Verification items for the finished model (mm, model axes). A direction names the side the tool comes from. Coordinates: 2 decimals unless noted, no trailing zeros. Write each loop counter-clockwise with the first axis right and the second up, starting at its lowest first coordinate (ties: lowest second). Pieces come first, ordered by that corner, then holes.
```python
from build123d import *

# Parameters (mm, degrees)
BOSS_EXTRUDE1_DEPTH = 1.7
BOSS_EXTRUDE4_DEPTH = 0.3
SKETCH6_R           = 1.45
CUT_EXTRUDE1_DEPTH  = 2
SKETCH7_R           = 1.45
CUT_EXTRUDE2_DEPTH  = 2
SKETCH8_R           = 0.25
CUT_EXTRUDE3_DEPTH  = 2
SKETCH9_R           = 0.25
CUT_EXTRUDE4_DEPTH  = 2


with BuildPart() as part:
    # Sketch1 → Boss-Extrude1 (new body)
    with BuildSketch(Plane.XY):
        Polygon((-93.349083219, 17.192602894), (-83.349083219, 17.192602894), (-83.349083219, 20.192602894), (-78.349083219, 20.192602894), (-78.349083219, 6.092602894), (-83.349083219, 6.092602894), (-83.349083219, 9.092602894), (-93.349083219, 9.092602894), (-93.349083219, 6.092602894), (-98.349083219, 6.092602894), (-98.349083219, 20.192602894), (-93.349083219, 20.192602894), align=None)
    extrude(amount=BOSS_EXTRUDE1_DEPTH)

    # Sketch1<4> → Boss-Extrude4 (add)
    with BuildSketch(Plane.XY):
        Polygon((-93.349083219, 17.192602894), (-83.349083219, 17.192602894), (-83.349083219, 20.192602894), (-78.349083219, 20.192602894), (-78.349083219, 6.092602894), (-83.349083219, 6.092602894), (-83.349083219, 9.092602894), (-93.349083219, 9.092602894), (-93.349083219, 6.092602894), (-98.349083219, 6.092602894), (-98.349083219, 20.192602894), (-93.349083219, 20.192602894), align=None)
    extrude(amount=-BOSS_EXTRUDE4_DEPTH)

    # Sketch6 → Cut-Extrude1 (cut)
    with BuildSketch(Plane.XY.offset(1.7)):
        with Locations((-95.349083219, 13.142602894)):
            Circle(SKETCH6_R)
    extrude(amount=-CUT_EXTRUDE1_DEPTH, mode=Mode.SUBTRACT)

    # Sketch7 → Cut-Extrude2 (cut)
    with BuildSketch(Plane.XY.offset(1.7)):
        with Locations((-90.349083219, 13.142602894)):
            Circle(SKETCH7_R)
    extrude(amount=-CUT_EXTRUDE2_DEPTH, mode=Mode.SUBTRACT)

    # Sketch8 → Cut-Extrude3 (cut)
    with BuildSketch(Plane.XY.offset(1.7)):
        with Locations((-83.349083219, 15.742602894)):
            Circle(SKETCH8_R)
    extrude(amount=-CUT_EXTRUDE3_DEPTH, mode=Mode.SUBTRACT)

    # Sketch9 → Cut-Extrude4 (cut)
    with BuildSketch(Plane.XY.offset(1.7)):
        with Locations((-83.349083219, 10.542602894)):
            Circle(SKETCH9_R)
    extrude(amount=-CUT_EXTRUDE4_DEPTH, mode=Mode.SUBTRACT)


solid = part.part
```
1. Tool access check on faces 1 (the flat face through (-83.349, 19, 1)), 2 (the flat face through (-93.349, 8, 1)), 3 (the flat face through (-96, 6.093, 1)). Record the directions out of +Z, -Z, +X, -X, +Y, -Y that give a thin tool (end or side, any length) a straight path to the whole face; none if there is none.
2. Sectioned sample at C-C, the plane y = 14. Record the boundary of the cut face in (x, z), and give its area (3 significant figures).
3. Gauge pin test, flat ends, axial feed: P1, Ø0.6, axis at x = -86.5, z = 0.5, coming from the +Y side; P2, Ø1, axis at x = -89, z = 0.5, coming from the -Y side. Record the tip position at first contact, or that the pin passes through.
4. Sectioned sample at D-D, the plane x = -84. Record the boundary of the cut face in (y, z), and give its area (3 significant figures).
5. Sectioned sample at A-A, the plane y = 17.75. Record the boundary of the cut face in (x, z), and give its area (3 significant figures).
6. Sectioned sample at B-B, the plane z = 0.1. Record the boundary of the cut face in (x, y).
7. Draft check along X on faces 4 (the flat face through (-88, 9.093, 1)), 5 (the flat face through (-98.349, 13, 1)), 6 (the flat face through (-88, 13, -0.3)). Enter one of: pulls with the +X half, pulls with the -X half, needs draft (parallel to the pull), parting line crosses it, or undercut.
8. Material ranges on L1, parallel to X at y = 13.25, z = 0.8; L2, parallel to X at y = 17.75, z = 1.4; L3, parallel to X at y = 14, z = 0.95, recorded low to high.
Outcome:
1. face 1: +Z, -Z, +Y
1. face 2: +Z, -Z, -Y
1. face 3: +Z, -Z, +X, -X, -Y
2. outline: (-98.35, -0.3) - (-96.52, -0.3) - (-96.52, 1.7) - (-98.35, 1.7) - close; (-94.18, -0.3) - (-91.52, -0.3) - (-91.52, 1.7) - (-94.18, 1.7) - close; (-89.18, -0.3) - (-78.35, -0.3) - (-78.35, 1.7) - (-89.18, 1.7) - close
2. area: 30.6 mm2
3. P1: stops at y = 17.19
3. P2: stops at y = 9.09
4. outline: (9.09, -0.3) - (17.19, -0.3) - (17.19, 1.7) - (9.09, 1.7) - close
4. area: 16.2 mm2
5. outline: (-98.35, -0.3) - (-93.35, -0.3) - (-93.35, 1.7) - (-98.35, 1.7) - close; (-83.35, -0.3) - (-78.35, -0.3) - (-78.35, 1.7) - (-83.35, 1.7) - close
5. area: 20.0 mm2
6. outline: (-98.35, 6.09) - (-93.35, 6.09) - (-93.35, 9.09) - (-83.35, 9.09) - (-83.35, 6.09) - (-78.35, 6.09) - (-78.35, 20.19) - (-83.35, 20.19) - (-83.35, 17.19) - (-93.35, 17.19) - (-93.35, 20.19) - (-98.35, 20.19) - close; hole circle Ø2.9 at (-95.35, 13.14); hole circle Ø2.9 at (-90.35, 13.14); hole circle Ø0.5 at (-83.35, 10.54); hole circle Ø0.5 at (-83.35, 15.74)
7. face 4: undercut
7. face 5: pulls with the -X half
7. face 6: needs draft
8. L1: x = -98.35 to -96.8, -93.9 to -91.8, -88.9 to -78.35
8. L2: x = -98.35 to -93.35, -83.35 to -78.35
8. L3: x = -98.35 to -96.52, -94.18 to -91.52, -89.18 to -78.35
